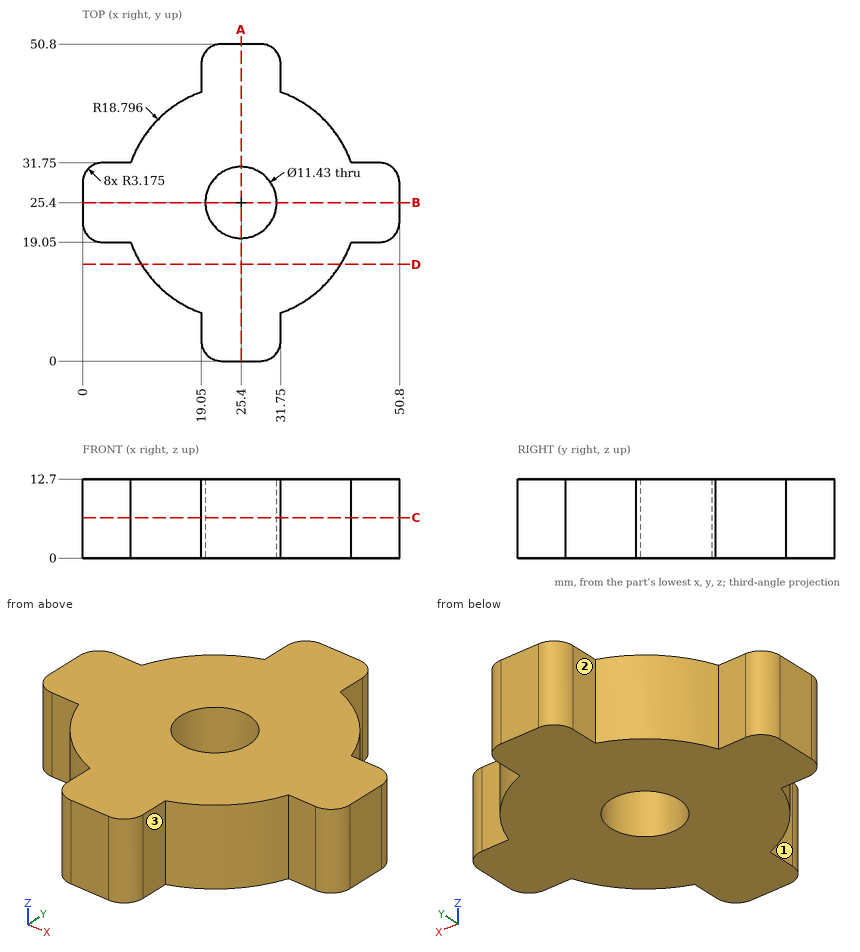
Part print with two shaded views. Sizes in mm from the minimum x, y, z corner. A direction names the side the tool comes from. Coordinates: 2 decimals unless noted, no trailing zeros. Write each loop counter-clockwise with the first axis right and the second up, starting at its lowest first coordinate (ties: lowest second). Pieces come first, ordered by that corner, then holes. Notation, with made-up numbers: (-6, 31) - (39, 31) arc R30 ccw to (39, 59) - close; hole circle Ø9 at (24, 30). An arc over 180 degrees is marked (long way). One line per item, written item: value. Start each with the question number.
1. Slice it at D-D (y = 15.5). Write the cut outline in (x, z).
2. Flat gauge pins, fed straight in: pin 1 (5 mm diameter, centred on x = 45, z = 6.5, fed in from -Y); pin 2 (2 mm diameter, centred on x = 12, z = 10.5, fed in from -Y); pin 3 (2.5 mm diameter, centred on x = 44.5, z = 8.5, fed in from +Y). Where does each tip first touch, or does it go through?
3. Tool access for the marked faces 1, 2 and 3: list every direction of +Z, -Z, +X, -X, +Y, -Y with a clear straight run to the whole face (end or side of a thin tool).
4. Probe line 1 (Y direction, x = 25.4, z = 5.5) (3 decimals); line 2 (Y direction, x = 24.5, z = 5); line 3 (X direction, y = 6.5, z = 4.25). List the from-to ranges inside material, lowest first. Write a range as from..to.
5. Slice it at A-A (x = 25.4). Write the cut outline in (y, z) (3 decimals), plus the area to 3 significant figures.
6. Slice it at C-C (z = 6.5). Write the cut outline in (x, y) (3 decimals).
Answers below:
1. outline: (9.42, 0) - (41.38, 0) - (41.38, 12.7) - (9.42, 12.7) - close
2. pin 1: stops at y = 17.6
2. pin 2: stops at y = 11.27
2. pin 3: stops at y = 31.75
3. face 1: +Z, -Z, -X, -Y
3. face 2: +Z, -Z, -X, +Y
3. face 3: +Z, -Z, +X, -Y
4. line 1: y = 0..19.685, 31.115..50.8
4. line 2: y = 0..19.76, 31.04..50.8
4. line 3: x = 19.05..31.75
5. outline: (0, 0) - (19.685, 0) - (19.685, 12.7) - (0, 12.7) - close; (31.115, 0) - (50.8, 0) - (50.8, 12.7) - (31.115, 12.7) - close
5. area: 500 mm^2
6. outline: (0, 22.225) arc R3.175 ccw to (3.175, 19.05) - (7.709, 19.05) arc R18.796 ccw to (19.05, 7.709) - (19.05, 3.175) arc R3.175 ccw to (22.225, 0) - (28.575, 0) arc R3.175 ccw to (31.75, 3.175) - (31.75, 7.709) arc R18.796 ccw to (43.091, 19.05) - (47.625, 19.05) arc R3.175 ccw to (50.8, 22.225) - (50.8, 28.575) arc R3.175 ccw to (47.625, 31.75) - (43.091, 31.75) arc R18.796 ccw to (31.75, 43.091) - (31.75, 47.625) arc R3.175 ccw to (28.575, 50.8) - (22.225, 50.8) arc R3.175 ccw to (19.05, 47.625) - (19.05, 43.091) arc R18.796 ccw to (7.709, 31.75) - (3.175, 31.75) arc R3.175 ccw to (0, 28.575) - close; hole circle Ø11.43 at (25.4, 25.4)
